CAD build for the part. Positions are in the model's coordinates, mm. Face numbers are marked on the shaded views. Round coordinates to 2 decimals unless told otherwise and drop trailing zeros. Order: outer loops, then holes, each group sorted by start corner. A loop starts at its lowest first (then second) coordinate and runs counter-clockwise, first axis right, second up. Notation, with made-up numbers: (87, 59.5) -> (123, 59.5) arc R13 ccw to (123, 79.5) -> close; hole circle Ø4 at (12, -36.5). An arc over 180 degrees is marked (long way). Return JSON: item names as keys, results as strings. Group by question number.
Q1. Probe line 1 along Z through (x, y) = (3, 1); line 2 along Y through (x, z) = (0, 9); line 3 along X through (y, z) = (-8, 15.5). List the from-to ranges inside material, lowest first.
Q2. Mould opens along Y. For the marked faces 1, 2 and 3 say: +Y half, -Y half, draft (parallel to the pull), parting line (faces both ways), or undercut.
Q3. Cut at D-D (z = 13.5). Write the cut outline in (x, y), then the cut area to 3 significant figures.
Q4. Cut at C-C (z = 22). Write the cut outline in (x, y), then the cut area to 3 significant figures.
Q5. Flat gauge pins, fed straight in: pin 1 (1 mm diameter, centred on y = 5.5, z = 4, fed in from +X); pin 2 (12 mm diameter, centred on x = 9.5, y = -7, fed in from +Z); pin 3 (10 mm diameter, centred on y = -3, z = 9.5, fed in from -X). Where does each tip first touch, or does it go through?
Q6. Cut at A-A (y = 0). Write the cut outline in (x, z).
from build123d import *

# Parameters (mm, degrees)
SKETCH1_R           = 23.25
SKETCH1_R_2         = 20.25
SKETCH1_R_3         = 17
BOSS_EXTRUDE1_DEPTH = 3
SKETCH1_3_R         = 23.25
SKETCH1_3_R_2       = 20.25
BOSS_EXTRUDE2_DEPTH = 35
SKETCH6_W           = 3
SKETCH6_H           = 3
CUT_EXTRUDE1_DEPTH  = 50.992661477


with BuildPart() as part:
    # Sketch1 → Boss-Extrude1 (new body)
    with BuildSketch(Plane.XY):
        Circle(SKETCH1_R)
        Circle(SKETCH1_R_2, mode=Mode.SUBTRACT)
        Circle(SKETCH1_R_2)
        Circle(SKETCH1_R_3, mode=Mode.SUBTRACT)
        Circle(SKETCH1_R_3)
    extrude(amount=-BOSS_EXTRUDE1_DEPTH)

    # Sketch1_3 → Boss-Extrude2 (add)
    with BuildSketch(Plane.XY):
        Circle(SKETCH1_3_R)
        Circle(SKETCH1_3_R_2, mode=Mode.SUBTRACT)
    extrude(amount=BOSS_EXTRUDE2_DEPTH)

    # Sketch4 → Revolve2 (revolve)
    with BuildSketch(Plane(origin=(0, 0, 0), x_dir=(1, 0, 0), z_dir=(0, 1, 0))):
        Polygon((23.25, -35), (23.25, 3), (25.241495613, -35), align=None)
    revolve(axis=Axis((0, 0, 0), (0, 0, 1)))

    # Sketch6 → Cut-Extrude1 (cut, through all)
    with BuildSketch(Plane.XY):
        with Locations((-10, 10)):
            Rectangle(SKETCH6_W, SKETCH6_H)
        with Locations((-5, 10)):
            Rectangle(SKETCH6_W, SKETCH6_H)
        with Locations((0, 10)):
            Rectangle(SKETCH6_W, SKETCH6_H)
        with Locations((5, 10)):
            Rectangle(SKETCH6_W, SKETCH6_H)
        with Locations((10, 10)):
            Rectangle(SKETCH6_W, SKETCH6_H)
        with Locations((10, 5)):
            Rectangle(SKETCH6_W, SKETCH6_H)
        with Locations((5, 5)):
            Rectangle(SKETCH6_W, SKETCH6_H)
        with Locations((0, 5)):
            Rectangle(SKETCH6_W, SKETCH6_H)
        with Locations((-5, 5)):
            Rectangle(SKETCH6_W, SKETCH6_H)
        with Locations((-10, 5)):
            Rectangle(SKETCH6_W, SKETCH6_H)
        with Locations((-10, 0)):
            Rectangle(SKETCH6_W, SKETCH6_H)
        with Locations((-10, -5)):
            Rectangle(SKETCH6_W, SKETCH6_H)
        with Locations((-5, 0)):
            Rectangle(SKETCH6_W, SKETCH6_H)
        with Locations((-5, -5)):
            Rectangle(SKETCH6_W, SKETCH6_H)
        Rectangle(SKETCH6_W, SKETCH6_H)
        with Locations((5, 0)):
            Rectangle(SKETCH6_W, SKETCH6_H)
        with Locations((10, 0)):
            Rectangle(SKETCH6_W, SKETCH6_H)
        with Locations((10, -5)):
            Rectangle(SKETCH6_W, SKETCH6_H)
        with Locations((5, -5)):
            Rectangle(SKETCH6_W, SKETCH6_H)
        with Locations((0, -5)):
            Rectangle(SKETCH6_W, SKETCH6_H)
        with Locations((-10, -10)):
            Rectangle(SKETCH6_W, SKETCH6_H)
        with Locations((-5, -10)):
            Rectangle(SKETCH6_W, SKETCH6_H)
        with Locations((0, -10)):
            Rectangle(SKETCH6_W, SKETCH6_H)
        with Locations((5, -10)):
            Rectangle(SKETCH6_W, SKETCH6_H)
        with Locations((10, -10)):
            Rectangle(SKETCH6_W, SKETCH6_H)
    extrude(amount=-CUT_EXTRUDE1_DEPTH, mode=Mode.SUBTRACT)


solid = part.part
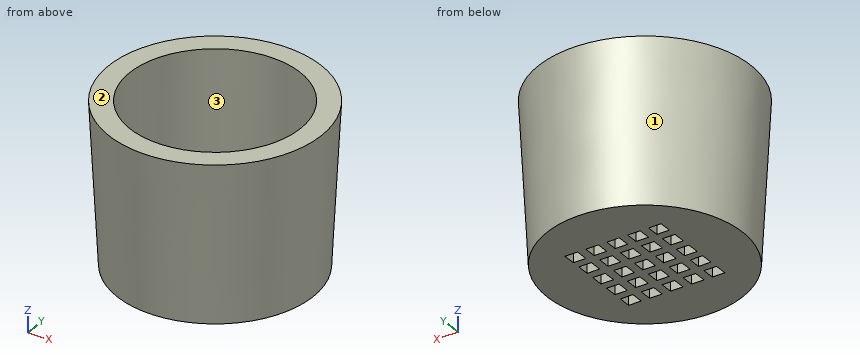
Solution:
{
 "1": {"line 1": "z = -3 to 0", "line 2": "y = -23.88 to -20.25, 20.25 to 23.88", "line 3": "x = -22.86 to -18.6, 18.6 to 22.86"},
 "2": {"face 1": "parting line", "face 2": "draft", "face 3": "undercut"},
 "3": {"outline": "circle Ø48.23 at (0, 0); hole circle Ø40.5 at (0, 0)", "area": "539 mm²"},
 "4": {"outline": "circle Ø49.12 at (0, 0); hole circle Ø40.5 at (0, 0)", "area": "607 mm²"},
 "5": {"pin 1": "stops at x = 23.08", "pin 2": "stops at z = 0", "pin 3": "stops at x = -24.13"},
 "6": {"outline": "(-25.24, 35) -> (-23.25, -3) -> (-11.5, -3) -> (-11.5, 0) -> (-20.25, 0) -> (-20.25, 35) -> close; (-8.5, -3) -> (-6.5, -3) -> (-6.5, 0) -> (-8.5, 0) -> close; (-3.5, -3) -> (-1.5, -3) -> (-1.5, 0) -> (-3.5, 0) -> close; (1.5, -3) -> (3.5, -3) -> (3.5, 0) -> (1.5, 0) -> close; (6.5, -3) -> (8.5, -3) -> (8.5, 0) -> (6.5, 0) -> close; (11.5, -3) -> (23.25, -3) -> (25.24, 35) -> (20.25, 35) -> (20.25, 0) -> (11.5, 0) -> close"}
}
